Drawing for the job (mm, zero at the part's lowest x, y, z). A direction names the side the tool comes from. Coordinates: 2 decimals unless noted, no trailing zeros. Loops run counter-clockwise (first coordinate to the right, second up) from the corner with the lowest first, then second, coordinate; pieces in that order, holes last. Notation, with made-up numbers: (-8.5, -22.5) - (19.5, -22.5) arc R17 ccw to (19.5, -1.5) - close; hole circle Ø5 at (2, -22.5). An arc over 180 degrees is marked (long way). One line per item, written item: value.
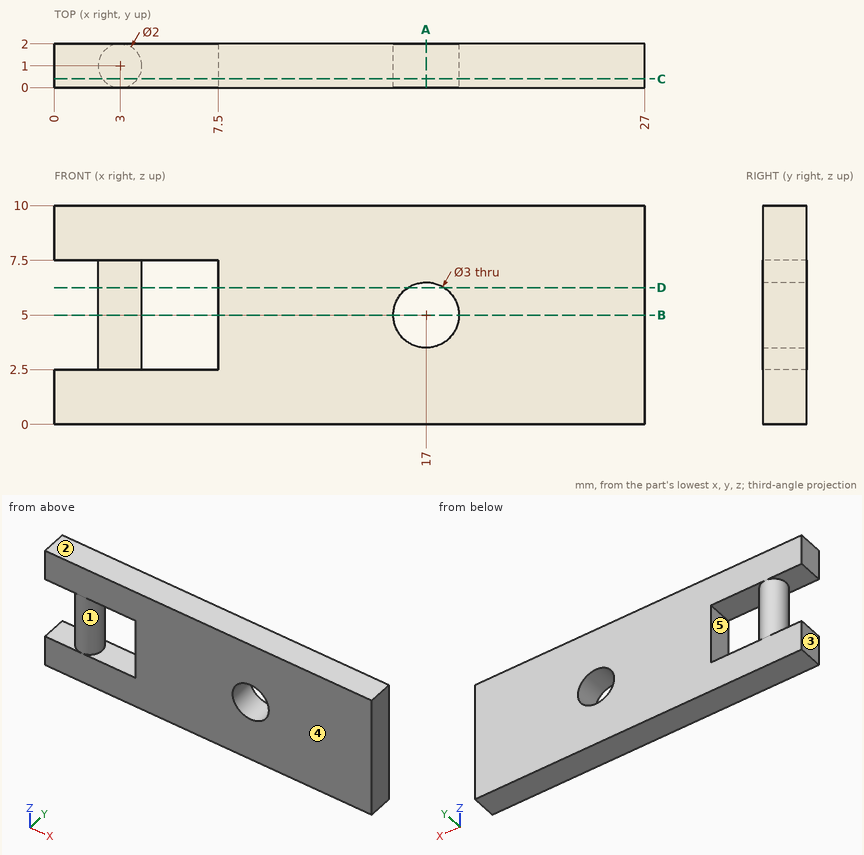
Item 1: Cut at C-C, the plane y = 0.4. Write the cut outline in (x, z), then the cut area to 3 significant figures.
Check result:
outline: (0, 0) - (27, 0) - (27, 10) - (0, 10) - (0, 7.5) - (2.2, 7.5) - (2.2, 2.5) - (0, 2.5) - close; hole (3.8, 2.5) - (7.5, 2.5) - (7.5, 7.5) - (3.8, 7.5) - close; hole circle Ø3 at (17, 5)
area: 233 mm^2
Item 2: Pull direction X, two halves, no side cores. Call the marked faces 1, 2 and 3: released by +X, released by -X, zero draft, split by the parting line, or undercut.
Check result:
face 1: undercut
face 2: zero draft
face 3: released by -X
Item 3: Probe probe 1 along X at (y, z) = (1.05, 5); probe 2 along Z at (x, y) = (6.75, 0.95); probe 3 along Z at (x, y) = (17, 0.9). List the from-to ranges inside material, lowest first. Write a range as from..to.
Check result:
probe 1: x = 2..4, 7.5..15.5, 18.5..27
probe 2: z = 0..2.5, 7.5..10
probe 3: z = 0..3.5, 6.5..10
Item 4: Cut at B-B, the plane z = 5. Write the cut outline in (x, y), then the cut area to 3 significant figures.
Check result:
outline: circle Ø2 at (3, 1); (7.5, 0) - (15.5, 0) - (15.5, 2) - (7.5, 2) - close; (18.5, 0) - (27, 0) - (27, 2) - (18.5, 2) - close
area: 36.1 mm^2
Item 5: Drop a flat-ended pin along its axis: P1, Ø1, axis at y = 1.5, z = 4.5, coming from the -X side. Give the stop position or say it passes through.
Check result:
P1: stops at x = 2
Item 6: Cut at A-A, the plane x = 17. Write the cut outline in (y, z), then the cut area to 3 significant figures.
Check result:
outline: (0, 0) - (2, 0) - (2, 3.5) - (0, 3.5) - close; (0, 6.5) - (2, 6.5) - (2, 10) - (0, 10) - close
area: 14.0 mm^2
Item 7: Tool access for the marked faces 4 and 5: list every direction of +Z, -Z, +X, -X, +Y, -Y with a clear straight run to the whole face (end or side of a thin tool).
Check result:
face 4: +Z, -Z, +X, -X, -Y
face 5: +Y, -Y
Item 8: Cut at D-D, the plane z = 6.25. Write the cut outline in (x, y).
Check result:
outline: circle Ø2 at (3, 1); (7.5, 0) - (16.17, 0) - (16.17, 2) - (7.5, 2) - close; (17.83, 0) - (27, 0) - (27, 2) - (17.83, 2) - close
